Study the drawing (mm; zero at the part's minimum x, y, z) and answer. Round coordinates to 2 decimals unless told otherwise and drop trailing zeros. Order: outer loops, then holes, each group sorted by start corner. A loop starts at its lowest first (then second) coordinate and runs counter-clockwise, first axis right, second up. Notation, with made-up numbers: (74, 34) - (126, 34) arc R37 cw to (126, 73) - close; hole circle Ø3 at (-13, -36). An arc over 180 degrees is marked (long way). Use one line per item in the form item = value. Start each with the question number.
Q1. Given P1, Ø5, axis at x = 8, y = 8, coming from the +Z side, flat-ended and moving along its own axis, determine where the tip first touches the part or whether it passes through.
Q2. The part is cut by section C-C on z = 0.2. Determine the outline of the cut face in (x, y).
Q3. The part is cut by section D-D on z = 1.3. Determine the outline of the cut face in (x, y).
Q4. For a pull along X with two mould halves and no side action, classify the marked faces 1 and 2 as +X half, -X half, draft (parallel to the pull), parting line (faces both ways), or undercut.
Q5. Find the intervals of material crossed by line 1 (Y direction, x = 8, z = 0.5); line 2 (X direction, y = 8.25, z = 0.7); line 3 (Y direction, x = 7, z = 0.7), in increasing order. Write a range as [from, to].
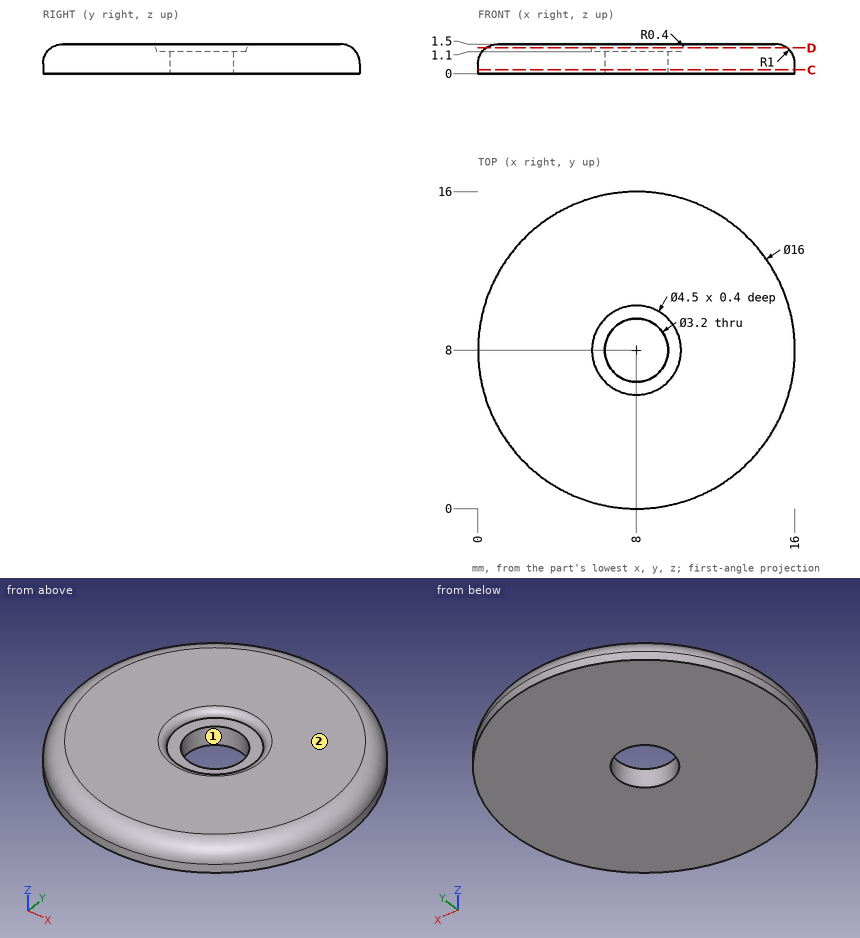
Found:
q1.P1 = 1.47
q2.outline = circle Ø16 at (8, 8); hole circle Ø3.2 at (8, 8)
q3.outline = circle Ø15.2 at (8, 8); hole circle Ø4.61 at (8, 8)
q4.face_1 = undercut
q4.face_2 = draft
q5.line_1 = [0, 6.4], [9.6, 16]
q5.line_2 = [0.02, 6.42], [9.58, 15.98]
q5.line_3 = [0.08, 6.75], [9.25, 15.92]
